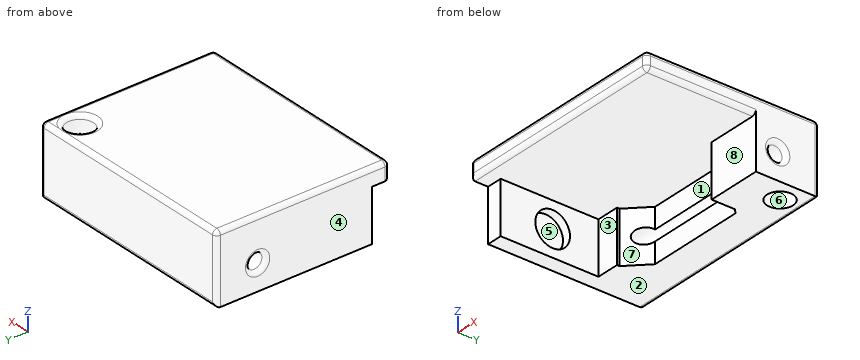
```python
from build123d import *

# Parameters (mm, degrees)
ESQUISSE1_W             = 25
ESQUISSE1_H             = 20
ESQUISSE1_R             = 1.55
BOSS_EXTRU_1_DEPTH      = 2
ESQUISSE2_R             = 1.5
BOSS_EXTRU_2_DEPTH      = 6
ESQUISSE3_R             = 2
ENL_V_MAT_EXTRU_1_DEPTH = 1
ESQUISSE4_R             = 0.9
ENL_V_MAT_EXTRU_2_DEPTH = 33.57299495
CONG_1_R                = 0.5
CONG_5_R                = 0.5
CONG_6_R                = 0.5


with BuildPart() as part:
    # Esquisse1 → Boss.-Extru.1 (new body)
    with BuildSketch(Plane.XY):
        with Locations((12.5, 10)):
            Rectangle(ESQUISSE1_W, ESQUISSE1_H)
        with Locations((22.5, 17.5)):
            Circle(ESQUISSE1_R, mode=Mode.SUBTRACT)
    extrude(amount=BOSS_EXTRU_1_DEPTH)

    # Esquisse2 → Boss.-Extru.2 (add)
    with BuildSketch(Plane(origin=(0, 0, 0), x_dir=(-1, 0, 0), z_dir=(0, 0, -1))):
        Polygon((-18.688890735, 12.684019913), (-18.688890735, 15.355693182), (-18.19165929, 15.852924628), (-6.705637613, 15.852924628), (-4.442134245, 13.58942126), (-4.442134245, 13.288407081), (-1.8, 13.288407081), (-1.8, 2), (0, 2), (0, 13.565515823), (0, 20), (-25, 20), (-25, 12.684019913), align=None)
        with Locations((-22.5, 17.5)):
            Circle(ESQUISSE2_R, mode=Mode.SUBTRACT)
    extrude(amount=BOSS_EXTRU_2_DEPTH)

    # Esquisse3 → Enlèv. mat.-Extru.1 (cut)
    with BuildSketch(Plane(origin=(1.8, 0, 0), x_dir=(0, 0, -1), z_dir=(1, 0, 0))):
        with Locations(Location((3, 8, 0), (0, 0, 90))):
            Circle(ESQUISSE3_R)
    extrude(amount=-ENL_V_MAT_EXTRU_1_DEPTH, mode=Mode.SUBTRACT)

    # Esquisse4 → Enlèv. mat.-Extru.2 (cut, through all)
    with BuildSketch(Plane.ZY):
        with Locations((-3, 15.2)):
            Circle(ESQUISSE4_R)
    extrude(amount=-ENL_V_MAT_EXTRU_2_DEPTH, mode=Mode.SUBTRACT)

    # Congé1
    # the kernel refuses this fillet: 0.5 mm, written as the material it takes off along each edge
    with BuildSketch(Plane(origin=(25, 15.2, -3), x_dir=(0, 0, 1), z_dir=(0, -1, 0))) as cong_1_piece_1:
        with BuildLine():
            CenterArc((0.9 + CONG_1_R, CONG_1_R), CONG_1_R, 180, 90)
            Line((0.9, CONG_1_R), (0.9, 0))
            Line((0.9, 0), (0.9 + CONG_1_R, 0))
        make_face()
    revolve(axis=Axis((25, 15.2, -3), (-1, 0, 0)), mode=Mode.SUBTRACT)
    with BuildSketch(Plane(origin=(18.688890735, 15.2, -3), x_dir=(0, 0.9999845857082649, -0.005552327968503009), z_dir=(0, 0.005552327968503009, 0.9999845857082649))) as cong_1_piece_2_section:
        with BuildLine():
            CenterArc((0.9 + CONG_1_R, -CONG_1_R), CONG_1_R, 90, 90)
            Line((0.9 + CONG_1_R, 0), (0.9, 0))
            Line((0.9, 0), (0.9, -CONG_1_R))
        make_face()
    cong_1_piece_2 = revolve(axis=Axis((18.688890735, 15.2, -3), (-1, 0, 0)), revolution_arc=269.681873406, mode=Mode.PRIVATE)
    cong_1_piece_2 = split(cong_1_piece_2, bisect_by=Plane(origin=(19.358402527, 14.68618139, -3.05957258), z_dir=(-0.7071067811865438, -0.7071067811865513, 0)), keep=Keep.TOP, mode=Mode.PRIVATE)
    add(cong_1_piece_2, mode=Mode.SUBTRACT)
    with BuildSketch(Plane(origin=(0, 15.2, -3), x_dir=(0, 0, 1), z_dir=(0, -1, 0))) as cong_1_piece_3:
        with BuildLine():
            CenterArc((0.9 + CONG_1_R, -CONG_1_R), CONG_1_R, 90, 90)
            Line((0.9, -CONG_1_R), (0.9, 0))
            Line((0.9, 0), (0.9 + CONG_1_R, 0))
        make_face()
    revolve(axis=Axis((0, 15.2, -3), (-1, 0, 0)), mode=Mode.SUBTRACT)
    with BuildSketch(Plane(origin=(18.688890735, 15.2, -3), x_dir=(0, 0, 1), z_dir=(0, -1, 0))) as cong_1_piece_4_section:
        with BuildLine():
            CenterArc((0.9 + CONG_1_R, -CONG_1_R), CONG_1_R, 90, 90)
            Line((0.9 + CONG_1_R, 0), (0.9, 0))
            Line((0.9, 0), (0.9, -CONG_1_R))
        make_face()
    cong_1_piece_4 = revolve(axis=Axis((18.688890735, 15.2, -3), (-1, 0, 0)), revolution_arc=89.539713829, mode=Mode.PRIVATE)
    cong_1_piece_4 = split(cong_1_piece_4, bisect_by=Plane(origin=(18.759427014, 15.285156904, -1.94281096), z_dir=(-0.7071067811865438, -0.7071067811865513, 0)), keep=Keep.TOP, mode=Mode.PRIVATE)
    add(cong_1_piece_4, mode=Mode.SUBTRACT)

    # Congé5
    # the kernel refuses this fillet: 0.5 mm, written as the material it takes off along each edge
    with BuildSketch(Plane(origin=(24.5, 0.5, 1.5), x_dir=(0, 0, 1), z_dir=(0, -1, 0))) as cong_5_piece_1_section:
        Polygon((0, 0), (CONG_5_R, 0), (CONG_5_R, -CONG_5_R), (0, -CONG_5_R), align=None)
    cong_5_piece_1 = extrude(amount=CONG_5_R, mode=Mode.PRIVATE)
    cong_5_piece_1 = cong_5_piece_1 - Plane(origin=(24.5, 0.5, 1.5), x_dir=(-0.7071067811865475, 0, -0.7071067811865475), z_dir=(0, -1, 0)) * Sphere(CONG_5_R, mode=Mode.PRIVATE)
    add(cong_5_piece_1, mode=Mode.SUBTRACT)
    with BuildSketch(Plane(origin=(24.5, 19.5, 1.5), x_dir=(1, 0, 0), z_dir=(0, 0, 1))) as cong_5_piece_2_section:
        Polygon((0, 0), (CONG_5_R, 0), (CONG_5_R, CONG_5_R), (0, CONG_5_R), align=None)
    cong_5_piece_2 = extrude(amount=CONG_5_R, mode=Mode.PRIVATE)
    cong_5_piece_2 = cong_5_piece_2 - Plane(origin=(24.5, 19.5, 1.5), x_dir=(-0.7071067811865475, -0.7071067811865475, 0), z_dir=(0, 0, 1)) * Sphere(CONG_5_R, mode=Mode.PRIVATE)
    add(cong_5_piece_2, mode=Mode.SUBTRACT)
    with BuildSketch(Plane(origin=(0.5, 19.5, 1.5), x_dir=(-1, 0, 0), z_dir=(0, 0, 1))) as cong_5_piece_3_section:
        Polygon((0, 0), (CONG_5_R, 0), (CONG_5_R, -CONG_5_R), (0, -CONG_5_R), align=None)
    cong_5_piece_3 = extrude(amount=CONG_5_R, mode=Mode.PRIVATE)
    cong_5_piece_3 = cong_5_piece_3 - Plane(origin=(0.5, 19.5, 1.5), x_dir=(0.7071067811865475, -0.7071067811865475, 0), z_dir=(0, 0, 1)) * Sphere(CONG_5_R, mode=Mode.PRIVATE)
    add(cong_5_piece_3, mode=Mode.SUBTRACT)
    with BuildSketch(Plane(origin=(0.5, 0.5, 1.5), x_dir=(0, 0, 1), z_dir=(0, -1, 0))) as cong_5_piece_4_section:
        Polygon((0, 0), (CONG_5_R, 0), (CONG_5_R, CONG_5_R), (0, CONG_5_R), align=None)
    cong_5_piece_4 = extrude(amount=CONG_5_R, mode=Mode.PRIVATE)
    cong_5_piece_4 = cong_5_piece_4 - Plane(origin=(0.5, 0.5, 1.5), x_dir=(0.7071067811865475, 0, -0.7071067811865475), z_dir=(0, -1, 0)) * Sphere(CONG_5_R, mode=Mode.PRIVATE)
    add(cong_5_piece_4, mode=Mode.SUBTRACT)
    with BuildSketch(Plane(origin=(22.5, 17.5, 2), x_dir=(1, 0, 0), z_dir=(0, -1, 0))) as cong_5_piece_5:
        with BuildLine():
            CenterArc((1.55 + CONG_5_R, -CONG_5_R), CONG_5_R, 90, 90)
            Line((1.55, -CONG_5_R), (1.55, 0))
            Line((1.55, 0), (1.55 + CONG_5_R, 0))
        make_face()
    revolve(axis=Axis((22.5, 17.5, 2), (0, 0, 1)), mode=Mode.SUBTRACT)
    with BuildSketch(Plane(origin=(25, 0.5, 2), x_dir=(-1, 0, 0), z_dir=(0, 1, 0)), Plane(origin=(0, 19.5, 2), x_dir=(1, 0, 0), z_dir=(0, -1, 0))) as cong_5_piece_6:
        with BuildLine():
            CenterArc((CONG_5_R, -CONG_5_R), CONG_5_R, 90, 90)
            Line((0, -CONG_5_R), (0, 0))
            Line((0, 0), (CONG_5_R, 0))
        make_face()
    extrude(amount=19, mode=Mode.SUBTRACT)
    with BuildSketch(Plane(origin=(24.5, 20, 2), x_dir=(0, -1, 0), z_dir=(-1, 0, 0))) as cong_5_piece_7:
        with BuildLine():
            CenterArc((CONG_5_R, -CONG_5_R), CONG_5_R, 90, 90)
            Line((0, -CONG_5_R), (0, 0))
            Line((0, 0), (CONG_5_R, 0))
        make_face()
    extrude(amount=24, mode=Mode.SUBTRACT)
    with BuildSketch(Plane(origin=(-1.25, 20, -6), x_dir=(0, -1, 0), z_dir=(1, 0, 0)), Plane(origin=(-1.25, 0, 0), x_dir=(0, 0, 1), z_dir=(1, 0, 0))) as cong_5_piece_8:
        with BuildLine():
            CenterArc((CONG_5_R, -CONG_5_R), CONG_5_R, 90, 90)
            Line((0, -CONG_5_R), (0, 0))
            Line((0, 0), (CONG_5_R, 0))
        make_face()
    extrude(amount=27.5, mode=Mode.SUBTRACT)
    with BuildSketch(Plane(origin=(0, 20, 1.5), x_dir=(1, 0, 0), z_dir=(0, 0, -1)), Plane(origin=(25, 20, -7.25), x_dir=(-1, 0, 0), z_dir=(0, 0, 1))) as cong_5_piece_9:
        with BuildLine():
            CenterArc((CONG_5_R, CONG_5_R), CONG_5_R, 180, 90)
            Line((0, CONG_5_R), (0, 0))
            Line((0, 0), (CONG_5_R, 0))
        make_face()
    extrude(amount=8.75, mode=Mode.SUBTRACT)
    with BuildSketch(Plane(origin=(25, 0, -1.25), x_dir=(-1, 0, 0), z_dir=(0, 0, 1))) as cong_5_piece_10:
        with BuildLine():
            CenterArc((CONG_5_R, -CONG_5_R), CONG_5_R, 90, 90)
            Line((0, -CONG_5_R), (0, 0))
            Line((0, 0), (CONG_5_R, 0))
        make_face()
    extrude(amount=2.75, mode=Mode.SUBTRACT)
    with BuildSketch(Plane(origin=(0, 0, -1.25), x_dir=(1, 0, 0), z_dir=(0, 0, 1))) as cong_5_piece_11:
        with BuildLine():
            CenterArc((CONG_5_R, CONG_5_R), CONG_5_R, 180, 90)
            Line((0, CONG_5_R), (0, 0))
            Line((0, 0), (CONG_5_R, 0))
        make_face()
    extrude(amount=2.75, mode=Mode.SUBTRACT)
    with BuildSketch(Plane(origin=(0.5, 0, 2), x_dir=(0, 0, -1), z_dir=(1, 0, 0))) as cong_5_piece_12:
        with BuildLine():
            CenterArc((CONG_5_R, CONG_5_R), CONG_5_R, 180, 90)
            Line((0, CONG_5_R), (0, 0))
            Line((0, 0), (CONG_5_R, 0))
        make_face()
    extrude(amount=24, mode=Mode.SUBTRACT)

    # Congé6
    # the kernel refuses this fillet: 0.5 mm, written as the material it takes off along each edge
    with BuildSketch(Plane(origin=(24.5, 0.5, 0.5), x_dir=(1, 0, 0), z_dir=(0, 0, -1))) as cong_6_piece_1_section:
        Polygon((0, 0), (CONG_6_R, 0), (CONG_6_R, CONG_6_R), (0, CONG_6_R), align=None)
    cong_6_piece_1 = extrude(amount=CONG_6_R, mode=Mode.PRIVATE)
    cong_6_piece_1 = cong_6_piece_1 - Plane(origin=(24.5, 0.5, 0.5), x_dir=(-0.7071067811865475, 0.7071067811865475, 0), z_dir=(0, 0, -1)) * Sphere(CONG_6_R, mode=Mode.PRIVATE)
    add(cong_6_piece_1, mode=Mode.SUBTRACT)
    with BuildSketch(Plane(origin=(25, 0.5, 0), x_dir=(-1, 0, 0), z_dir=(0, 1, 0))) as cong_6_piece_2:
        with BuildLine():
            CenterArc((CONG_6_R, CONG_6_R), CONG_6_R, 180, 90)
            Line((0, CONG_6_R), (0, 0))
            Line((0, 0), (CONG_6_R, 0))
        make_face()
    extrude(amount=12.184019913, mode=Mode.SUBTRACT)


solid = part.part
```
Verification items for the finished model (mm, model axes). Face numbers are marked on the shaded views. A direction names the side the tool comes from. Coordinates: 2 decimals unless noted, no trailing zeros. Write each loop counter-clockwise with the first axis right and the second up, starting at its lowest first coordinate (ties: lowest second). Pieces come first, ordered by that corner, then holes. Notation, with made-up numbers: (11, 42.5) - (41, 42.5) arc R18 ccw to (41, 71.5) - close; hole circle Ø5 at (32, -34.75). An arc over 180 degrees is marked (long way). One line per question, with ' | ' between items. Start each with the question number.
1. Draft check along X on the marked faces 1, 2, 3 and 4. Enter one of: released by +X, released by -X, zero draft, split by the parting line, or undercut.
2. Section check A-A (x = 10.75). Enter the section's corners in (y, z), plus the area to 3 significant figures.
3. Section check B-B (z = -3). Enter the section's corners in (x, y).
4. Section check C-C (y = 12). Enter the section's corners in (x, z).
5. Gauge pin test, flat ends, axial feed: P1, Ø3, axis at y = 8.5, z = -2.5, coming from the +X side; P2, Ø2.5, axis at x = 22.5, y = 17.5, coming from the -Z side; P3, Ø0.7, axis at x = 9.5, z = -4.5, coming from the -Y side; P4, Ø2.5, axis at x = 23, y = 17, coming from the +Z side. Record the tip position at first contact, or that the pin passes through.
6. Access from +Z, -Z, +X, -X, +Y, -Y to the whole of each face (thin tool, end or side, straight path). Record for the marked faces 5, 6, 7 and 8.
7. Section check D-D (x = 5). Enter the section's corners in (y, z).
8. Material ranges on line 1 along Y through (x, z) = (22.5, 1.2); line 2 along Y through (x, z) = (15.25, -3); line 3 along Z through (x, y) = (1.45, 8), recorded low to high.
Computed values:
1) face 1: undercut | face 2: zero draft | face 3: undercut | face 4: released by -X
2) outline: (0, 0.5) arc R0.5 ccw to (0.5, 0) - (15.85, 0) - (15.85, -2.38) arc R0.9 cw to (15.85, -3.62) - (15.85, -6) - (19.5, -6) arc R0.5 ccw to (20, -5.5) - (20, 1.5) arc R0.5 ccw to (19.5, 2) - (0.5, 2) arc R0.5 ccw to (0, 1.5) - close | area: 64.5 mm²
3) outline: (0, 2) - (1.8, 2) - (1.8, 6) - (0.8, 6) - (0.8, 10) - (1.8, 10) - (1.8, 13.29) - (4.44, 13.29) - (4.44, 13.59) - (5.15, 14.3) - (0.5, 14.3) arc R0.5 ccw to (0, 13.8) - close; (0, 16.6) arc R0.5 ccw to (0.5, 16.1) - (21.96, 16.1) arc R1.5 cw (long way) to (23.04, 16.1) - (24.5, 16.1) arc R0.5 ccw to (25, 16.6) - (25, 19.5) arc R0.5 ccw to (24.5, 20) - (0.5, 20) arc R0.5 ccw to (0, 19.5) - close; (18.69, 12.68) - (25, 12.68) - (25, 13.8) arc R0.5 ccw to (24.5, 14.3) - (19.19, 14.3) arc R0.5 ccw to (18.69, 13.8) - close
4) outline: (0, -6) - (1.8, -6) - (1.8, 0) - (24.5, 0) arc R0.5 ccw to (25, 0.5) - (25, 1.5) arc R0.5 ccw to (24.5, 2) - (0.5, 2) arc R0.5 ccw to (0, 1.5) - close
5) P1: x = 1.8 | P2: through | P3: y = 15.85 | P4: z = 1.99
6) face 5: +X | face 6: +Z, -Z | face 7: -Z, -Y | face 8: -Z, +X, -Y
7) outline: (0, 0.5) arc R0.5 ccw to (0.5, 0) - (14.15, 0) - (14.15, -6) - (19.5, -6) arc R0.5 ccw to (20, -5.5) - (20, 1.5) arc R0.5 ccw to (19.5, 2) - (0.5, 2) arc R0.5 ccw to (0, 1.5) - close; hole circle Ø1.8 at (15.2, -3)
8) line 1: 0 to 15.95, 19.05 to 20 | line 2: 16.1 to 20 | line 3: -6 to -5, -1 to 2
